The figure shows three views and two pictorial views of one solid part (mm, origin at its lowest corner). Answer the questions. A direction names the side the tool comes from. Coordinates: 2 decimals unless noted, no trailing zeros. Write each loop counter-clockwise with the first axis right and the second up, starting at its lowest first coordinate (ties: lowest second). Pieces come first, ordered by that corner, then holes. Notation, with made-up numbers: M 79,79 L 91,79 A11 ccw 91,83 Z; hole C 69.25,36 d1. An arc over 180 degrees is marked long. Write item = value, one per line.
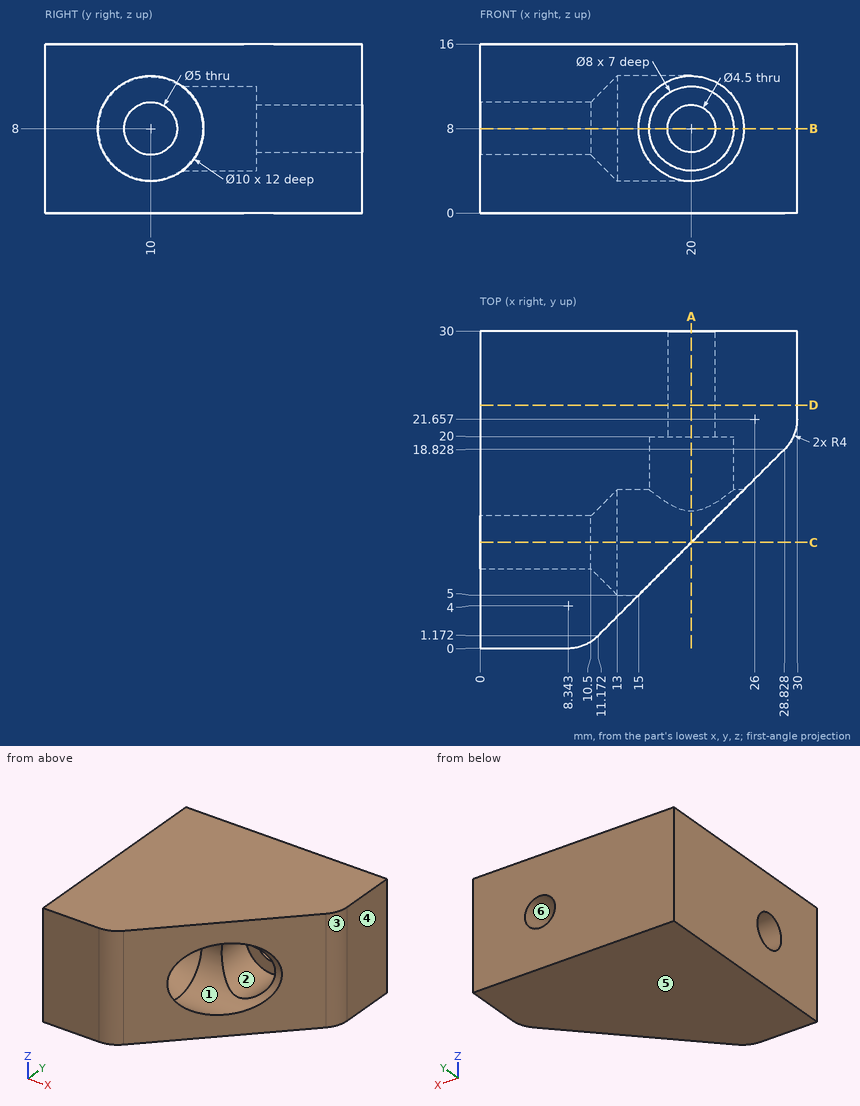
Item 1: A flat-ended cylindrical pin translates along its axis: pin 1 (5 mm diameter, centred on x = 11, z = 10, fed in from -Y). Find the tip coordinate at first contact, or state that the pin passes through.
Worked answers:
pin_1 = 0
Item 2: Which of the six approach directions +Z, -Z, +X, -X, +Y, -Y give full straight-line access (tool end or side, diameter ignored) to the marked faces 1, 2 and 3?
Worked answers:
face_1 = +X
face_2 = -Y
face_3 = +Z, -Z, +X, -Y
Item 3: For a pull along Z with two mould halves and no side action, classify the marked faces 4, 5 and 6 as released by +Z, released by -Z, zero draft, split by the parting line, or undercut.
Worked answers:
face_4 = zero draft
face_5 = released by -Z
face_6 = undercut
Item 4: Find section B-B (z = 8). Determine the outline of the cut face in (x, y), and give its area (3 significant figures).
Worked answers:
outline = M 0,0 L 8.34,0 A4 ccw 11.17,1.17 L 15,5 L 13,5 L 10.5,7.5 L 0,7.5 Z; M 0,12.5 L 10.5,12.5 L 13,15 L 16,15 L 16,20 L 17.75,20 L 17.75,30 L 0,30 Z; M 22.25,20 L 24,20 L 24,15 L 25,15 L 28.83,18.83 A4 ccw 30,21.66 L 30,30 L 22.25,30 Z
area = 473 mm²
Item 5: Find section A-A (x = 20). Determine the outline of the cut face in (y, z), and give its area (3 significant figures).
Worked answers:
outline = M 10,0 L 30,0 L 30,5.75 L 20,5.75 L 20,4 L 13,4 A5 cw 10,3 Z; M 10,13 A5 cw 13,12 L 20,12 L 20,10.25 L 30,10.25 L 30,16 L 10,16 Z
area = 191 mm²
Item 6: Consider line 1 along Z through (x, y) = (20, 22.25); line 2 along Z through (x, y) = (19, 17.25); line 3 along Y through (x, z) = (1, 6.75) (1 decimal). Determine where each line is inside the solid, lowest interval first. Write a range as from..to.
Worked answers:
line_1 = 0..5.75, 10.25..16
line_2 = 0..4.13, 11.87..16
line_3 = 0..7.8, 12.2..30
Item 7: Find section D-D (y = 23). Determine the outline of the cut face in (x, z), and give its area (3 significant figures).
Worked answers:
outline = M 0,0 L 30,0 L 30,16 L 0,16 Z; hole C 20,8 d4.5
area = 464 mm²
Item 8: Find section C-C (y = 10). Determine the outline of the cut face in (x, z), and give its area (3 significant figures).
Worked answers:
outline = M 0,0 L 20,0 L 20,3 L 13,3 L 10.5,5.5 L 0,5.5 Z; M 0,10.5 L 10.5,10.5 L 13,13 L 20,13 L 20,16 L 0,16 Z
area = 179 mm²
